Design review of the part built by this model. Coordinates are the model's own, in mm. A direction names the side the tool comes from. Round coordinates to 2 decimals unless told otherwise and drop trailing zeros. Order: outer loops, then holes, each group sorted by start corner. A loop starts at its lowest first (then second) coordinate and runs counter-clockwise, first axis right, second up. Notation, with made-up numbers: (-31, 3) - (-7, 3) arc R27 ccw to (-7, 30) - close; hole circle Ø11 at (0, -38). An arc over 180 degrees is marked (long way). Use CSV: the item, a comma, the result in double quotes.
from build123d import *

# Parameters (mm, degrees)
SKETCH1_W           = 37
SKETCH1_H           = 62
SKETCH1_R           = 1.15
BOSS_EXTRUDE1_DEPTH = 1.2
SKETCH2_W           = 31.928778657
SKETCH2_H           = 49.046896963
BOSS_EXTRUDE2_DEPTH = 2
SKETCH3_R           = 0.75
CUT_EXTRUDE1_DEPTH  = 73.228803119


with BuildPart() as part:
    # Sketch1 → Boss-Extrude1 (new body)
    with BuildSketch(Plane(origin=(0, 0, 0), x_dir=(1, 0, 0), z_dir=(0, 1, 0))):
        with Locations((18.5, 31)):
            Rectangle(SKETCH1_W, SKETCH1_H)
        with Locations(Location((32.5, 60, 0), (0, 0, 270))):
            Circle(SKETCH1_R, mode=Mode.SUBTRACT)
        with Locations(Location((4.5, 60, 0), (0, 0, 270))):
            Circle(SKETCH1_R, mode=Mode.SUBTRACT)
        with Locations(Location((32.5, 2, 0), (0, 0, 270))):
            Circle(SKETCH1_R, mode=Mode.SUBTRACT)
        with Locations(Location((4.5, 2, 0), (0, 0, 270))):
            Circle(SKETCH1_R, mode=Mode.SUBTRACT)
    extrude(amount=BOSS_EXTRUDE1_DEPTH)

    # Sketch2 → Boss-Extrude2 (add)
    with BuildSketch(Plane(origin=(0, 1.2, 0), x_dir=(1, 0, 0), z_dir=(0, 1, 0))):
        with Locations((18.2105599, 31.643941755)):
            Rectangle(SKETCH2_W, SKETCH2_H)
    extrude(amount=BOSS_EXTRUDE2_DEPTH)

    # Sketch3 → Cut-Extrude1 (cut, through all)
    with BuildSketch(Plane(origin=(0, 1.2, 0), x_dir=(1, 0, 0), z_dir=(0, 1, 0))):
        with Locations(Location((9.031578358, 2.050688375, 0), (0, 0, 270))):
            Circle(SKETCH3_R)
        with Locations(Location((11.531578358, 2.050688375, 0), (0, 0, 270))):
            Circle(SKETCH3_R)
        with Locations(Location((14.031578358, 2.050688375, 0), (0, 0, 270))):
            Circle(SKETCH3_R)
        with Locations(Location((16.531578358, 2.050688375, 0), (0, 0, 270))):
            Circle(SKETCH3_R)
        with Locations(Location((19.031578358, 2.050688375, 0), (0, 0, 270))):
            Circle(SKETCH3_R)
        with Locations(Location((21.531578358, 2.050688375, 0), (0, 0, 270))):
            Circle(SKETCH3_R)
        with Locations(Location((24.031578358, 2.050688375, 0), (0, 0, 270))):
            Circle(SKETCH3_R)
        with Locations(Location((26.531578358, 2.050688375, 0), (0, 0, 270))):
            Circle(SKETCH3_R)
    extrude(amount=-CUT_EXTRUDE1_DEPTH, mode=Mode.SUBTRACT)


solid = part.part
1) For faces 1 (the face through (18, 2, -7.12)), 2 (the face through (18, 3.2, -32)), 3 (the face through (34.175, 2, -31)), list the 3-axis set-ups (+Z, -Z, +X, -X, +Y, -Y) from which the entire face can be reached by the end or side of a thin tool; tool diameter is ignored.
Data:
face 1,"+Z, +X, -X, +Y"
face 2,"+Z, -Z, +X, -X, +Y"
face 3,"+Z, -Z, +X, +Y"
2) We need section D-D (y = 1.95). Give the boundary of the cut face in (x, z), then the cut area to 3 significant figures.
Data:
outline,"(2.25, -56.17) - (34.17, -56.17) - (34.17, -7.12) - (2.25, -7.12) - close"
area,"1,570 mm2"
3) Insertion check: pin 1 Ø2 at (x, z) = (11.53, -2.05) entering from +Y; pin 2 Ø8 at (x, z) = (6, -48.5) entering from -Y; pin 3 Ø1.8 at (x, z) = (32.5, -2) entering from -Y; pin 4 Ø0.6 at (x, y) = (21.5, 2) entering from +Z. Each pin has a flat end and moves straight along its axis. Give the tip position at first contact, or say it passes through.
Data:
pin 1,"stops at y = 1.2"
pin 2,"stops at y = 0"
pin 3,"passes through"
pin 4,"stops at z = -7.12"
4) We need section B-B (x = 32.5). Give the boundary of the cut face in (y, z).
Data:
outline,"(0, -62) - (1.2, -62) - (1.2, -61.15) - (0, -61.15) - close; (0, -58.85) - (1.2, -58.85) - (1.2, -56.17) - (3.2, -56.17) - (3.2, -7.12) - (1.2, -7.12) - (1.2, -3.15) - (0, -3.15) - close; (0, -0.85) - (1.2, -0.85) - (1.2, 0) - (0, 0) - close"
5) We need section C-C (z = -30.5). Give the boundary of the cut face in (x, y).
Data:
outline,"(0, 0) - (37, 0) - (37, 1.2) - (34.17, 1.2) - (34.17, 3.2) - (2.25, 3.2) - (2.25, 1.2) - (0, 1.2) - close"
6) The part is to be moulded in two halves that separate along Z. For faces 4 (the face through (9.54, 0.61, -2.6)), 5 (the face through (18, 2, -56.167)), 6 (the face through (2.246, 2, -31)), say which applies: +Z half, -Z half, draft (parallel to the pull), parting line (faces both ways), or undercut.
Data:
face 4,"undercut"
face 5,"-Z half"
face 6,"draft"
7) To check wall thickness, follow L1, parallel to X at y = 0.6, z = -60; L2, parallel to Y at x = 10.5, z = -3; L3, parallel to Z at x = 8, y = 2.15. State the ranges of each line that lie inside material, in increasing order. Write a range as from..to.
Data:
L1,"x = 0..3.35, 5.65..31.35, 33.65..37"
L2,"y = 0..1.2"
L3,"z = -56.17..-7.12"
8) We need section A-A (z = -60). Give the boundary of the cut face in (x, y).
Data:
outline,"(0, 0) - (3.35, 0) - (3.35, 1.2) - (0, 1.2) - close; (5.65, 0) - (31.35, 0) - (31.35, 1.2) - (5.65, 1.2) - close; (33.65, 0) - (37, 0) - (37, 1.2) - (33.65, 1.2) - close"
